Design review of the part built by this model. Coordinates are the model's own, in mm. A direction names the side the tool comes from. Coordinates: 2 decimals unless noted, no trailing zeros. Write each loop counter-clockwise with the first axis right and the second up, starting at its lowest first coordinate (ties: lowest second). Pieces come first, ordered by that corner, then holes. Notation, with made-up numbers: (69, -17) - (110, -17) arc R9 ccw to (110, -12) - close; hole circle Ø8 at (-8, -28). An arc over 180 degrees is marked (long way). Answer as CSV lines item,"result". Start each with the question number.
Q1. For line 1 along X through (y, z) = (0, -344); line 2 along Z through (x, y) = (231.5, 1.75); line 3 along Y through (x, z) = (228, -353.5), list the stretches that pass through material, from the lowest coordinate up. Write a range as [from, to].
Q2. We need section A-A (z = -345.75). Write out the cut boundary in (x, y), plus the area to 3 significant figures.
Q3. We need section B-B (x = 199). Write out the cut boundary in (y, z).
Q4. Machinability: for faces 1 (the face through (299, 0, -351)), 2 (the face through (240, 0, -351)), 3 (the face through (184, 0, -346)), 4 (the face through (239, 7, -354)), which of the approach directions +Z, -Z, +X, -X, +Y, -Y give a long, thin tool a straight path to every point of the face, cutting with its end or side? Answer none if there is none.
Q5. Clearance check with flat-ended pins moving along their axes: pin 1 (5 mm diameter, centred on y = 3.5, z = -344.5, fed in from -X); pin 2 (1.8 mm diameter, centred on x = 298.5, y = -3, fed in from +Z); pin 3 (5.5 mm diameter, centred on x = 232.5, z = -354, fed in from -Y). State where each tip first meets the part, or that it passes through.
Q6. Mouldability with a two-part tool opening along X and no side actions: class faces 5 (the face through (239, -7, -354)), 6 (the face through (178, 0, -354)), 7 (the face through (302, 0, -354)), 8 (the face through (274, 0, -346)) as pulls with the +X half, pulls with the -X half, needs draft (parallel to the pull), parting line crosses it, or undercut.
Q7. We need section D-D (z = -352.5). Write out the cut boundary in (x, y), plus the area to 3 significant figures.
Q8. We need section C-C (y = 0.5). Write out the cut boundary in (x, z), plus the area to 3 significant figures.
from build123d import *

# Parameters (mm, degrees)
EXTRUDE_START      = -356
EXTRUDE_SKETCH_1_W = 124
EXTRUDE_SKETCH_1_H = 14
EXTRUDE_1_DEPTH    = 5
EXTRUDE_START_2    = -351
EXTRUDE_SKETCH_2_W = 22
EXTRUDE_SKETCH_2_H = 16
EXTRUDE_2_DEPTH    = 9.5
EXTRUDE_SKETCH_3_W = 22
EXTRUDE_SKETCH_3_H = 16
EXTRUDE_3_DEPTH    = 9.5


with BuildPart() as part:
    # Extrude sketch 1 → Extrude 1 (new body)
    with BuildSketch(Plane.XY.offset(EXTRUDE_START)):
        with Locations((240, 0)):
            Rectangle(EXTRUDE_SKETCH_1_W, EXTRUDE_SKETCH_1_H)
    extrude(amount=EXTRUDE_1_DEPTH)


with BuildPart() as body_2:
    # Extrude sketch 2 → Extrude 2 (new body)
    with BuildSketch(Plane.XY.offset(EXTRUDE_START_2)):
        with Locations((285, 0)):
            Rectangle(EXTRUDE_SKETCH_2_W, EXTRUDE_SKETCH_2_H)
    extrude(amount=EXTRUDE_2_DEPTH)


with BuildPart() as body_3:
    # Extrude sketch 3 → Extrude 3 (new body)
    with BuildSketch(Plane.XY.offset(EXTRUDE_START_2)):
        with Locations((195, 0)):
            Rectangle(EXTRUDE_SKETCH_3_W, EXTRUDE_SKETCH_3_H)
    extrude(amount=EXTRUDE_3_DEPTH)


with BuildPart() as part_1:
    add(part.part)

    # Combine (weld / assembly of features): union body 2, body 3
    add(body_2.part)
    add(body_3.part)


solid = part_1.part
Results list:
1,line 1,"x = [184, 206], [274, 296]"
1,line 2,"z = [-356, -351]"
1,line 3,"y = [-7, 7]"
2,outline,"(184, -8) - (206, -8) - (206, 8) - (184, 8) - close; (274, -8) - (296, -8) - (296, 8) - (274, 8) - close"
2,area,"704 mm2"
3,outline,"(-8, -351) - (-7, -351) - (-7, -356) - (7, -356) - (7, -351) - (8, -351) - (8, -341.5) - (-8, -341.5) - close"
4,face 1,"+Z, +X, +Y, -Y"
4,face 2,"+Z, +Y, -Y"
4,face 3,"+Z, -X, +Y, -Y"
4,face 4,"-Z, +X, -X, +Y"
5,pin 1,"stops at x = 184"
5,pin 2,"stops at z = -351"
5,pin 3,"stops at y = -7"
6,face 5,"needs draft"
6,face 6,"pulls with the -X half"
6,face 7,"pulls with the +X half"
6,face 8,"undercut"
7,outline,"(178, -7) - (302, -7) - (302, 7) - (178, 7) - close"
7,area,"1,740 mm2"
8,outline,"(178, -356) - (302, -356) - (302, -351) - (296, -351) - (296, -341.5) - (274, -341.5) - (274, -351) - (206, -351) - (206, -341.5) - (184, -341.5) - (184, -351) - (178, -351) - close"
8,area,"1,040 mm2"
